Build history of the part. All positions in model axes, mm. Face numbers are marked on the shaded views. A direction names the side the tool comes from. Coordinates: 2 decimals unless noted, no trailing zeros. Write each loop counter-clockwise with the first axis right and the second up, starting at its lowest first coordinate (ties: lowest second). Pieces come first, ordered by that corner, then holes.
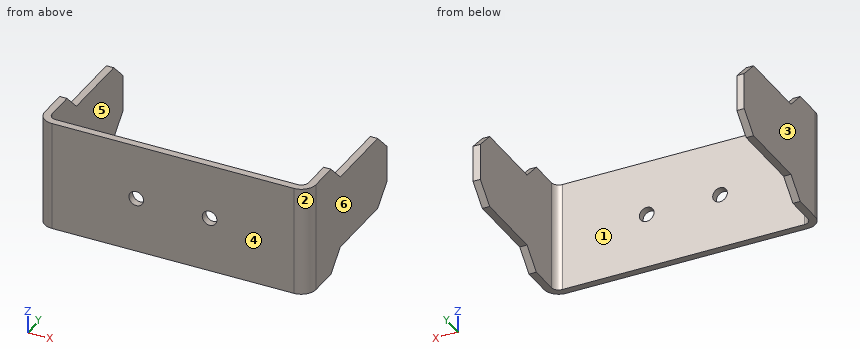
```python
from build123d import *

# Parameters (mm, degrees)
SKETCH_1_W               = 70
SKETCH_1_H               = 30
EXTRUDE_1_DEPTH          = 40
SHEET_START              = -15
SHEET_METAL_1_DEPTH      = 30
SHEET_METAL_1_2_DEPTH    = 30
CUT_EXTRUDE_1_REACH      = 58.515
SKETCH_6_R               = 2
CUT_EXTRUDE_3_DEPTH      = 57.515484604
CUT_EXTRUDE_3_DEPTH_BACK = 57.515484604
CHAMFER_1_SIZE           = 5


# Read off the part's stored shape, not the designer's step: 转换实体1
with BuildPart() as part:
    # Sketch 1 → 凸台-拉伸1 (new body)
    with BuildSketch(Plane(origin=(0, 0, 0), x_dir=(1, 0, 0), z_dir=(0, 1, 0))):
        Rectangle(SKETCH_1_W, SKETCH_1_H)
    extrude(amount=EXTRUDE_1_DEPTH)

    # Sheet Metal 1 outline → Sheet Metal 1 (cut)
    with BuildSketch(Plane.XY.offset(SHEET_START)):
        with BuildLine():
            Line((35, 2), (35, 40))
            Line((35, 40), (-35, 40))
            Line((-35, 40), (-35, 2))
            ThreePointArc((-35, 2), (-34.414213562, 0.585786438), (-33, 0))
            Line((-33, 0), (33, 0))
            ThreePointArc((33, 0), (34.414213562, 0.585786438), (35, 2))
        make_face()
    extrude(amount=SHEET_METAL_1_DEPTH, mode=Mode.SUBTRACT)

    # Sheet Metal 1 2 outline → Sheet Metal 1 2 (add)
    with BuildSketch(Plane.XY.offset(SHEET_START)):
        with BuildLine():
            Line((37, 2), (37, 40))
            Line((37, 40), (35, 40))
            Line((35, 40), (35, 0))
            Line((35, 0), (-35, 0))
            Line((-35, 0), (-35, 40))
            Line((-35, 40), (-37, 40))
            Line((-37, 40), (-37, 2))
            ThreePointArc((-37, 2), (-35.828427125, -0.828427125), (-33, -2))
            Line((-33, -2), (33, -2))
            ThreePointArc((33, -2), (35.828427125, -0.828427125), (37, 2))
        make_face()
    extrude(amount=SHEET_METAL_1_2_DEPTH)

    # 草图6 → 切除-拉伸1 (cut, up to next)
    with BuildSketch(Plane(origin=(0, 0, 0), x_dir=(1, 0, 0), z_dir=(0, 1, 0)), mode=Mode.PRIVATE) as cut_extrude_1_sk1:
        with Locations(Location((-10, 0, 0), (0, 0, 270))):
            Circle(SKETCH_6_R)
    cut_extrude_1_tool1 = extrude(cut_extrude_1_sk1.sketch, amount=-CUT_EXTRUDE_1_REACH, mode=Mode.PRIVATE) & part.part
    # 草图6 → 切除-拉伸1 (cut, up to next)
    with BuildSketch(Plane(origin=(0, 0, 0), x_dir=(1, 0, 0), z_dir=(0, 1, 0)), mode=Mode.PRIVATE) as cut_extrude_1_sk2:
        with Locations(Location((10, 0, 0), (0, 0, 270))):
            Circle(SKETCH_6_R)
    cut_extrude_1_tool2 = extrude(cut_extrude_1_sk2.sketch, amount=-CUT_EXTRUDE_1_REACH, mode=Mode.PRIVATE) & part.part
    add(cut_extrude_1_tool1.solids().sort_by_distance((-10, 0, 0))[0], mode=Mode.SUBTRACT)
    add(cut_extrude_1_tool2.solids().sort_by_distance((10, 0, 0))[0], mode=Mode.SUBTRACT)

    # 草图7 → 切除-拉伸3 (cut, two sides: drawn at the far end of the back side and taken through both)
    with BuildSketch(Plane(origin=(0, 0, 0), x_dir=(0, 0, -1), z_dir=(1, 0, 0)).offset(-CUT_EXTRUDE_3_DEPTH_BACK)):
        Polygon((-15, 10), (-10, 15), (-10, 40), (-15, 40), align=None)
        Polygon((10, 15), (10, 40), (15, 40), (15, 10), align=None)
    extrude(amount=CUT_EXTRUDE_3_DEPTH + CUT_EXTRUDE_3_DEPTH_BACK, mode=Mode.SUBTRACT)

    # 倒角1
    chamfer_1_edges = [part.edges().sort_by_distance(p)[0] for p in [
        (-36, 40, 10),
        (36, 40, 10),
        (-36, 40, -10),
        (36, 40, -10),
    ]]
    chamfer(chamfer_1_edges, length=CHAMFER_1_SIZE)


solid = part.part
```
1. Saw through at B-B on x = 10. List the corners of the cut face in (y, z).
Computed values:
outline: (-2, -15) - (0, -15) - (0, -2) - (-2, -2) - close; (-2, 2) - (0, 2) - (0, 15) - (-2, 15) - close
2. Mould opens along X. For the marked faces 1, 2, 3 and 4 say: +X half, -X half, draft (parallel to the pull), parting line (faces both ways), or undercut.
Computed values:
face 1: undercut
face 2: +X half
face 3: -X half
face 4: draft
3. 3-axis set-ups, long thin cutter, end or side, ignore diameter. For the marked faces 5 and 6: which of +Z, -Z, +X, -X, +Y, -Y reach the whole face in a straight line?
Computed values:
face 5: +Z, -Z, +Y
face 6: +Z, -Z, +X, +Y, -Y
4. Saw through at A-A on y = 9. List the corners of the cut face in (x, z), plus the area to 3 significant figures.
Computed values:
outline: (-37, -15) - (-35, -15) - (-35, 15) - (-37, 15) - close; (35, -15) - (37, -15) - (37, 15) - (35, 15) - close
area: 120 mm2
5. Saw through at C-C on z = 0. List the corners of the cut face in (x, y).
Computed values:
outline: (-37, 2) arc R4 ccw to (-33, -2) - (-12, -2) - (-12, 0) - (-33, 0) arc R2 cw to (-35, 2) - (-35, 40) - (-37, 40) - close; (-8, -2) - (8, -2) - (8, 0) - (-8, 0) - close; (12, -2) - (33, -2) arc R4 ccw to (37, 2) - (37, 40) - (35, 40) - (35, 2) arc R2 cw to (33, 0) - (12, 0) - close
6. Flat gauge pins, fed straight in: pin 1 (2 mm diameter, centred on x = -35.5, y = 26.5, fed in from +Z); pin 2 (2 mm diameter, centred on x = 36, y = 28, fed in from -Z); pin 3 (1.5 mm diameter, centred on x = 16.5, z = 5, fed in from +Y); pin 4 (6.5 mm diameter, centred on x = -10, z = 0, fed in from -Y). Where does each tip first touch, or does it go through?
Computed values:
pin 1: stops at z = 10
pin 2: stops at z = -10
pin 3: stops at y = 0
pin 4: stops at y = -2
7. Probe line 1 along X through (y, z) = (-0.65, 0); line 2 along X through (y, z) = (-1.3, 0); line 3 along X through (y, z) = (11, -5.5). List the from-to ranges inside material, lowest first.
Computed values:
line 1: x = -36 to -12, -8 to 8, 12 to 36
line 2: x = -35.26 to -12, -8 to 8, 12 to 35.26
line 3: x = -37 to -35, 35 to 37
8. Saw through at D-D on z = 12.5. List the corners of the cut face in (x, y).
Computed values:
outline: (-37, 2) arc R4 ccw to (-33, -2) - (33, -2) arc R4 ccw to (37, 2) - (37, 12.5) - (35, 12.5) - (35, 2) arc R2 cw to (33, 0) - (-33, 0) arc R2 cw to (-35, 2) - (-35, 12.5) - (-37, 12.5) - close
